from build123d import *

# Parameters (mm, degrees)
PAD_DEPTH        = 6
HOLE_D           = 3
HOLE_CBORE_D     = 4.5
HOLE_CBORE_DEPTH = 25
CHAMFER_SIZE     = 0.6
FILLET_R         = 20


with BuildPart() as part:
    # Sketch → Pad (new body)
    with BuildSketch(Plane.XY):
        with BuildLine():
            ThreePointArc((26.398653, -9.333333), (0, 28), (-26.398653, -9.333333))
            ThreePointArc((-30.169889, -10.666667), (-27.617605, -11.885618), (-26.398653, -9.333333))
            ThreePointArc((-25, 19.974984), (-31.554031, 5.323827), (-30.169889, -10.666667))
            Line((-25, 19.974984), (-25, 35))
            Line((-25, 35), (25, 35))
            Line((25, 19.974984), (25, 35))
            ThreePointArc((30.169889, -10.666667), (31.554031, 5.323827), (25, 19.974984))
            ThreePointArc((26.398653, -9.333333), (27.617605, -11.885618), (30.169889, -10.666667))
        make_face()
    extrude(amount=PAD_DEPTH)

    # Hole (through all)
    with Locations(Plane.XZ):
        with Locations((-20, 3), (20, 3)):
            CounterBoreHole(HOLE_D / 2, HOLE_CBORE_D / 2, HOLE_CBORE_DEPTH)

    # Chamfer
    chamfer_edges = [part.edges().sort_by_distance(p)[0] for p in [
        (21.5, 25, 3),
        (-18.5, 25, 3),
    ]]
    chamfer(chamfer_edges, length=CHAMFER_SIZE)

    # Fillet
    fillet_edges = [part.edges().sort_by_distance(p)[0] for p in [
        (-25, 19.974984, 3),
        (25, 19.974984, 3),
    ]]
    fillet(fillet_edges, radius=FILLET_R)


solid = part.part
Could you check a few things on this model? Use its own coordinates, in mm. A direction names the side the tool comes from. Round coordinates to 2 decimals unless told otherwise and drop trailing zeros. Write each loop counter-clockwise with the first axis right and the second up, starting at its lowest first coordinate (ties: lowest second). Pieces come first, ordered by that corner, then holes. Notation, with made-up numbers: (-36.75, 44) - (-9.75, 44) arc R23 cw to (-9.75, 67) - close; hole circle Ø4 at (74, 72). An arc over 180 degrees is marked (long way). Put each result on its own line as item: value. Start each with the question number.
(1) I want a section at C-C, the plane x = 20. Please give me the cut outline in (y, z), plus the area to 3 significant figures.
(2) I need wall thicknesses on probe 1 along X at (y, z) = (30.5, 2); probe 2 along Z at (x, y) = (20, 27.5); probe 3 along X at (y, z) = (0, 2.5). Which ranges of each line are inside material? Lowest first, please.
(3) I want a section at D-D, the plane z = 3. Give the number of separate pieces and of enclosed holes in the cut face, plus the area to 3 significant figures.
(4) Will these pins go through, and if not, where does the flat tip stop? pin 1 (6 mm diameter, centred on x = 11.5, y = 19, fed in from -Z) (3 decimals); pin 2 (1.3 mm diameter, centred on x = -20, z = 2, fed in from -Y); pin 3 (1.5 mm diameter, centred on x = 16, y = 25, fed in from -Z); pin 4 (3 mm diameter, centred on y = 27.5, z = 2, fed in from -X).
(5) For faces 1 (the cylindrical face through (-22.248, 21.832, 3.099)), 2 (the flat face through (25, 30, 3)), 3 (the flat face through (-25, 30, 3)), which set-ups out of +Z, -Z, +X, -X, +Y, -Y let a thin tool reach every point of the face, with its end or its side?
(6) I want a section at B-B, the plane y = 31. Please give me the cut outline in (x, z).
(7) Thinking about a two-plate mould opening in Z: for faces 4 (the cylindrical face through (-18.5, 30.37, 3.07)), 5 (the cylindrical face through (-27.66, -11.9, 2.96)), 6 (the flat face through (-2, 29, 0)), 7 (the flat face through (-2, 29, 6)), which applies, released by +Z, released by -Z, zero draft, split by the parting line, or undercut?
(8) I want a section at A-A, the plane y = 0. Please give me the cut outline in (x, z).
Here are the results:
1. outline: (19.6, 0) - (35, 0) - (35, 1.5) - (25.6, 1.5) - (25, 0.9) - (25, 0.75) - (19.6, 0.75) - close; (19.6, 5.25) - (25, 5.25) - (25, 5.1) - (25.6, 4.5) - (35, 4.5) - (35, 6) - (19.6, 6) - close
1. area: 37.7 mm^2
2. probe 1: x = -25 to -21.12, -18.88 to 18.88, 21.12 to 25
2. probe 2: z = 0 to 1.5, 4.5 to 6
2. probe 3: x = -32 to -28, 28 to 32
3. separate pieces: 3
3. enclosed holes: 0
3. area: 700 mm^2
4. pin 1: passes through
4. pin 2: stops at y = 25.45
4. pin 3: stops at z = 0
4. pin 4: stops at x = -25
5. face 1: -Y
5. face 2: +Z, -Z, +X, +Y
5. face 3: +Z, -Z, -X, +Y
6. outline: (-25, 0) - (25, 0) - (25, 6) - (-25, 6) - close; hole circle Ø3 at (-20, 3); hole circle Ø3 at (20, 3)
7. face 4: undercut
7. face 5: zero draft
7. face 6: released by -Z
7. face 7: released by +Z
8. outline: (-32, 0) - (-28, 0) - (-28, 6) - (-32, 6) - close; (28, 0) - (32, 0) - (32, 6) - (28, 6) - close
